```python
from build123d import *

# Parameters (mm, degrees)
F0_R     = 0.75
F1_DEPTH = 20
F2_R     = 0.3
F3_DEPTH = 3
F4_R     = 0.15
F5_DEPTH = 7
F6_R     = 0.45
F7_DEPTH = 3
F8_R     = 0.25
F9_DEPTH = 7


with BuildPart() as f1:
    # F0 (on Top) → F1 (new body)
    with BuildSketch(Plane.XY):
        Circle(F0_R)
    extrude(amount=F1_DEPTH)

    # F2 (on face) → F3 (cut)
    with BuildSketch(Plane.XY.offset(20)):
        Circle(F2_R)
    extrude(amount=-F3_DEPTH, mode=Mode.SUBTRACT)

    # F4 (on face) → F5 (cut)
    with BuildSketch(Plane.XY.offset(17)):
        Circle(F4_R)
    extrude(amount=-F5_DEPTH, mode=Mode.SUBTRACT)

    # F6 (on face) → F7 (cut)
    with BuildSketch(Plane(origin=(0, 0, 0), x_dir=(1, 0, 0), z_dir=(0, 0, -1))):
        Circle(F6_R)
    extrude(amount=-F7_DEPTH, mode=Mode.SUBTRACT)

    # F8 (on face) → F9 (cut)
    with BuildSketch(Plane(origin=(0, 0, 3), x_dir=(1, 0, 0), z_dir=(0, 0, -1))):
        Circle(F8_R)
    extrude(amount=-F9_DEPTH, mode=Mode.SUBTRACT)


solid = f1.part
```
Geometry: final body of the model. Coordinates: model frame, mm. Give positions to 0.01 mm unless a question says otherwise; leave off trailing zeros. Order: outer loops, then holes, each group sorted by start corner. A loop starts at its lowest first (then second) coordinate and runs counter-clockwise, first axis right, second up. Notation, with made-up numbers: M -33.75,-11.75 L 3.25,-11.75 A16 cw 3.25,12.25 Z; hole C -32,87 d7. An arc over 180 degrees is marked long. Answer as CSV lines item,"result". Start each with the question number.
1) Cut plane B-B (z = 2.25). Output: boundary loops of the cut face in (x, y), then the cut area to 3 significant figures.
2) Cut plane A-A (z = 8.25). Output: boundary loops of the cut face in (x, y).
3) Line query: line 1 (Y direction, x = 0, z = 0.95); line 2 (Y direction, x = 0, z = 12.25); line 3 (Z direction, x = 0.15, y = 0.1). Output: solid intervals per line, ascending. Write a range as from..to.
4) First-contact query: P1, Ø0.6, axis at x = 0, y = 0, coming from the -Z side. Flat tip, straight axial feed; report the tip coordinate or a pass-through.
5) Mould query, pull axis Y, two halves, no side actions, for faces 1 (the cylindrical face through (0.429, -0.135, 1.479)), 2 (the cylindrical face through (-0.75, 0.03, 9.86)). Classes: +Y half, -Y half, draft (parallel to the pull), parting line (faces both ways), or undercut.
Findings below:
1,outline,"C 0,0 d1.5; hole C 0,0 d0.9"
1,area,"1.13 mm²"
2,outline,"C 0,0 d1.5; hole C 0,0 d0.5"
3,line 1,"y = -0.75..-0.45, 0.45..0.75"
3,line 2,"y = -0.75..-0.15, 0.15..0.75"
3,line 3,"z = 10..17"
4,P1,"stops at z = 3"
5,face 1,"undercut"
5,face 2,"parting line"
